from build123d import *

# Parameters (mm, degrees)
EXTRUDE_1_DEPTH          = 3
SKETCH_2_OUTSIDE_W       = 13.724
SKETCH_2_OUTSIDE_H       = 8.024
CUT_EXTRUDE_1_DEPTH      = 12
SKETCH_3_R               = 1.05
CUT_EXTRUDE_2_DEPTH      = 12
SKETCH_4_R               = 0.95
EXTRUDE_2_DEPTH          = 4
EXTRUDE_3_DEPTH          = 8
SKETCH_6_R               = 1.05
CUT_EXTRUDE_3_DEPTH      = 12
SKETCH_8_W               = 8
SKETCH_8_H               = 7
CUT_EXTRUDE_4_DEPTH      = 8
EXTRUDE_5_DEPTH          = 2
SKETCH_12_W              = 8
SKETCH_12_H              = 3
EXTRUDE_8_DEPTH          = 4
SKETCH_14_W              = 12
SKETCH_14_H              = 3
EXTRUDE_9_DEPTH          = 5
SKETCH_16_R              = 0.6
CUT_EXTRUDE_5_DEPTH      = 4
SKETCH_15_R              = 0.85
CUT_EXTRUDE_6_DEPTH      = 4
EXTRUDE_START            = 1.5
SKETCH_18_W              = 12
SKETCH_18_H              = 5.023607379
EXTRUDE_11_DEPTH         = 6
SKETCH_19_R              = 1.55
CUT_EXTRUDE_7_DEPTH      = 19.553975315
FILLET_1_R               = 1
CUT_EXTRUDE_8_DEPTH      = 19.553975315
CUT_EXTRUDE_8_DEPTH_BACK = 19.553975315
SKETCH_11_R              = 1.05
CUT_EXTRUDE_9_DEPTH      = 19.553975315
FILLET_2_R               = 1
SKETCH_21_W              = 8
SKETCH_21_H              = 2.221688244
CUT_EXTRUDE_10_DEPTH     = 12.939765268


with BuildPart() as part:
    # 草图1 → 凸台-拉伸1 (new body)
    with BuildSketch(Plane(origin=(0, 0, 0), x_dir=(1, 0, 0), z_dir=(0, 1, 0))):
        Polygon((-6, 0), (6, 0), (6, -8.7), (4, -8.7), (4, -3), (-4, -3), (-4, -8.7), (-6, -8.7), align=None)
    extrude(amount=EXTRUDE_1_DEPTH)

    # 草图2 outside → 切除-拉伸1 (cut)
    with BuildSketch(Plane.ZY.offset(6)):
        with Locations((4.35, 1.5)):
            Rectangle(SKETCH_2_OUTSIDE_W, SKETCH_2_OUTSIDE_H)
        with BuildLine():
            Line((6.2, 3), (0, 3))
            Line((0, 3), (0, 0))
            Line((0, 0), (6.2, 0))
            ThreePointArc((6.2, 0), (7.7, 1.5), (6.2, 3))
        make_face(mode=Mode.SUBTRACT)
    extrude(amount=-CUT_EXTRUDE_1_DEPTH, mode=Mode.SUBTRACT)

    # 草图3 → 切除-拉伸2 (cut)
    with BuildSketch(Plane.ZY.offset(6)):
        with Locations((5.2, 1.5)):
            Circle(SKETCH_3_R)
    extrude(amount=-CUT_EXTRUDE_2_DEPTH, mode=Mode.SUBTRACT)

    # 草图4 → 凸台-拉伸2 (add)
    with BuildSketch(Plane(origin=(0, 0, 0), x_dir=(-1, 0, 0), z_dir=(0, 0, -1))):
        with Locations((0, 1.5)):
            Circle(SKETCH_4_R)
    extrude(amount=EXTRUDE_2_DEPTH)

    # 草图5 → 凸台-拉伸3 (add)
    with BuildSketch(Plane(origin=(0, 0, -4), x_dir=(-1, 0, 0), z_dir=(0, 0, -1))):
        Polygon((-5, 3), (-6, 3), (-6, 0), (-4, 0), (4, 0), (6, 0), (6, 3), (5, 3), align=None)
    extrude(amount=EXTRUDE_3_DEPTH)

    # 草图6 → 切除-拉伸3 (cut)
    with BuildSketch(Plane(origin=(6, 0, 0), x_dir=(0, 0, -1), z_dir=(1, 0, 0))):
        with Locations((7.5, 1.5)):
            Circle(SKETCH_6_R)
    extrude(amount=-CUT_EXTRUDE_3_DEPTH, mode=Mode.SUBTRACT)

    # 草图8 → 切除-拉伸4 (cut)
    with BuildSketch(Plane(origin=(0, 3, 0), x_dir=(1, 0, 0), z_dir=(0, 1, 0))):
        with Locations((0, 8.5)):
            Rectangle(SKETCH_8_W, SKETCH_8_H)
    extrude(amount=-CUT_EXTRUDE_4_DEPTH, mode=Mode.SUBTRACT)

    # 草图10 → 凸台-拉伸5 (add)
    with BuildSketch(Plane.ZY.offset(6)):
        with BuildLine():
            Line((-12, 3), (-12, 5.5))
            ThreePointArc((-12, 5.5), (-10, 7.5), (-8, 5.5))
            Line((-8, 5.5), (-8, 3))
            Line((-8, 3), (-12, 3))
        make_face()
    extrude_5 = extrude(amount=-EXTRUDE_5_DEPTH)

    # 镜向1: 凸台-拉伸5 across plane
    add(extrude_5.mirror(Plane(origin=(0, 0, 0), x_dir=(0, 0, 1), z_dir=(1, 0, 0))))

    # 草图12 → 凸台-拉伸8 (add)
    with BuildSketch(Plane.XY.offset(-4)):
        with Locations((0, 1.5)):
            Rectangle(SKETCH_12_W, SKETCH_12_H)
    extrude(amount=EXTRUDE_8_DEPTH)

    # 草图14 → 凸台-拉伸9 (add)
    with BuildSketch(Plane(origin=(0, 0, 0), x_dir=(-1, 0, 0), z_dir=(0, 0, -1))):
        with Locations((0, 1.5)):
            Rectangle(SKETCH_14_W, SKETCH_14_H)
    extrude(amount=EXTRUDE_9_DEPTH)

    # 草图16 → 切除-拉伸5 (cut)
    with BuildSketch(Plane.ZY.offset(6)):
        with Locations((1.2, 1.5)):
            Circle(SKETCH_16_R)
    extrude(amount=-CUT_EXTRUDE_5_DEPTH, mode=Mode.SUBTRACT)

    # 草图15 → 切除-拉伸6 (cut)
    with BuildSketch(Plane(origin=(6, 0, 0), x_dir=(0, 0, -1), z_dir=(1, 0, 0))):
        with Locations((-1.2, 1.5)):
            Circle(SKETCH_15_R)
    extrude(amount=-CUT_EXTRUDE_6_DEPTH, mode=Mode.SUBTRACT)

    # 草图18 → 凸台-拉伸11 (add)
    with BuildSketch(Plane(origin=(0, 3, 0), x_dir=(1, 0, 0), z_dir=(0, 1, 0)).offset(EXTRUDE_START)):
        with Locations((0, -0.488196311)):
            Rectangle(SKETCH_18_W, SKETCH_18_H)
    extrude(amount=-EXTRUDE_11_DEPTH)

    # 草图19 → 切除-拉伸7 (cut, through all)
    with BuildSketch(Plane(origin=(6, 0, 0), x_dir=(0, 0, -1), z_dir=(1, 0, 0))):
        with Locations((-0.5, 1.5)):
            Circle(SKETCH_19_R)
    extrude(amount=-CUT_EXTRUDE_7_DEPTH, mode=Mode.SUBTRACT)

    # 圆角1
    fillet_1_edges = [part.edges().sort_by_distance(p)[0] for p in [
        (0, -1.5, -2.023607379),
        (0, -1.5, 3),
        (0, 4.5, 3),
        (0, 4.5, -2.023607379),
    ]]
    fillet(fillet_1_edges, radius=FILLET_1_R)

    # 草图11 → 切除-拉伸8 (cut, two sides: drawn at the far end of the back side and taken through both)
    with BuildSketch(Plane.ZY.offset(6).offset(-CUT_EXTRUDE_8_DEPTH_BACK)):
        with Locations((-10, 5.5)):
            Circle(SKETCH_11_R)
    extrude(amount=CUT_EXTRUDE_8_DEPTH + CUT_EXTRUDE_8_DEPTH_BACK, mode=Mode.SUBTRACT)

    # 草图20 → 切除-拉伸9 (cut, through all)
    with BuildSketch(Plane(origin=(6, 0, 0), x_dir=(0, 0, -1), z_dir=(1, 0, 0))):
        Polygon((8, 3), (9.290209613, 3), (9.290209613, 0), (12, 0), (12, 7.886253168), (8, 7.886253168), align=None)
    extrude(amount=-CUT_EXTRUDE_9_DEPTH, mode=Mode.SUBTRACT)

    # 圆角2
    fillet_2_edges = [part.edges().sort_by_distance(p)[0] for p in [
        (5, 0, -9.290209613),
        (-5, 0, -9.290209613),
        (5, 3, -9.290209613),
        (-5, 3, -9.290209613),
    ]]
    fillet(fillet_2_edges, radius=FILLET_2_R)

    # 草图21 → 切除-拉伸10 (cut, through all)
    with BuildSketch(Plane(origin=(0, 3, 0), x_dir=(1, 0, 0), z_dir=(0, 1, 0))):
        with Locations((0, 3.889155878)):
            Rectangle(SKETCH_21_W, SKETCH_21_H)
    extrude(amount=-CUT_EXTRUDE_10_DEPTH, mode=Mode.SUBTRACT)


solid = part.part
Part model, mm, in its own coordinate system. A direction names the side the tool comes from. Coordinates: 2 decimals unless noted, no trailing zeros. Order: outer loops, then holes, each group sorted by start corner. A loop starts at its lowest first (then second) coordinate and runs counter-clockwise, first axis right, second up.
(1) Slice it at D-D, the plane x = 2. Write the cut outline in (y, z).
Check sheet entries:
outline: (-1.5, -1.02) arc R1 ccw to (-0.5, -2.02) - (0, -2.02) - (0, -2.78) - (3, -2.78) - (3, -2.02) - (3.5, -2.02) arc R1 ccw to (4.5, -1.02) - (4.5, 2) arc R1 ccw to (3.5, 3) - (-0.5, 3) arc R1 ccw to (-1.5, 2) - close; hole circle Ø3.1 at (1.5, 0.5)
(2) Pull direction X, two halves, no side cores. Call faces 1 (the face through (4, 1, 4)), 2 (the face through (5, 0, 5)): pulls with the +X half, pulls with the -X half, needs draft (parallel to the pull), parting line crosses it, or undercut.
Check sheet entries:
face 1: undercut
face 2: needs draft
(3) Tool access for faces 3 (the face through (1.4, 0, -2.3)), 4 (the face through (5, 3, 5)), 5 (the face through (-4, 2, 4)), 6 (the face through (-5, 0, 5)): list every direction of +Z, -Z, +X, -X, +Y, -Y with a clear straight run to the whole face (end or side of a thin tool).
Check sheet entries:
face 3: -Z, +X, -X, -Y
face 4: +Z, +X, -X, +Y
face 5: +Z, +Y, -Y
face 6: +Z, +X, -X, -Y
(4) Slice it at A-A, the plane z = 5.2. Write the cut outline in (x, y), and give its area (3 significant figures).
Check sheet entries:
outline: (-6, 0) - (-4, 0) - (-4, 0.45) - (-6, 0.45) - close; (-6, 2.55) - (-4, 2.55) - (-4, 3) - (-6, 3) - close; (4, 0) - (6, 0) - (6, 0.45) - (4, 0.45) - close; (4, 2.55) - (6, 2.55) - (6, 3) - (4, 3) - close
area: 3.60 mm2
(5) Pin check, flat tips, straight feed: pin 1 Ø1 at (x, z) = (-5.5, 5) entering from -Y; pin 2 Ø1.2 at (x, y) = (-2.5, 1) entering from +Z; pin 3 Ø7 at (x, z) = (-1, -5) entering from +Y. Stop position of each tip, or through.
Check sheet entries:
pin 1: stops at y = 0
pin 2: stops at z = 3
pin 3: stops at y = 4.38
(6) Slice it at B-B, the plane y = 1.5. State how many separate pieces and enclosed holes the cut face has, and give its area (3 significant figures).
Check sheet entries:
separate pieces: 6
enclosed holes: 0
area: 60.2 mm2
(7) Probe L1, parallel to X at y = 1.2, z = 4; L2, parallel to Y at x = 0.5, z = 0.5; L3, parallel to Z at x = 4.75, y = 1.7. List the from-to ranges inside material, lowest first.
Check sheet entries:
L1: x = -6 to -4, 4 to 6
L2: y = -1.5 to -0.05, 3.05 to 4.5
L3: z = -9.29 to -8.53, -6.47 to -1.04, 2.04 to 4.17, 6.23 to 7.69
(8) Slice it at C-C, the plane z = -6. Write the cut outline in (x, y).
Check sheet entries:
outline: (-6, 0) - (-4, 0) - (-4, 3) - (-6, 3) - close; (4, 0) - (6, 0) - (6, 3) - (4, 3) - close
